Source: three-view drawing plus pictorial views. Frame: mm from the lowest corner of the part. Give positions to 0.01 mm unless a question says otherwise; leave off trailing zeros. Order: outer loops, then holes, each group sorted by start corner. A loop starts at its lowest first (then second) coordinate and runs counter-clockwise, first axis right, second up. Notation, with made-up numbers: (66.5, 85.25) -> (74.5, 85.25) arc R25 cw to (74.5, 120.25) -> close; hole circle Ø4 at (14, 84.5). An arc over 180 degrees is marked (long way). Answer in a Markdown table with one row per item. Add a question column.
Q1. Pull-direction query (X, two-part tool) for the marked faces 1, 2 and 3; classes: +X half, -X half, draft (parallel to the pull), parting line (faces both ways), or undercut.
Q2. Cut plane A-A on z = 40. Return the cut outline in (x, y).
Q3. Line query: line 1 along X through (y, z) = (2.8, 40); line 2 along X through (y, z) = (22, 40). Output: solid intervals per line, ascending. Write a range as from..to.
Q4. Cut plane C-C on y = 10.5. Return the cut outline in (x, z), and give its area (3 significant figures).
Q5. Cut plane B-B on x = 40. Return the cut outline in (y, z), and give its area (3 significant figures).
Q6. Cut plane D-D on x = 29.5. Return the cut outline in (y, z), and give its area (3 significant figures).
Q7. Contact query for flat-ended pins moving along their axis: P1, Ø5, axis at x = 55.5, y = 9.5, coming from the +Z side; P2, Ø2, axis at x = 49.5, y = 31, coming from the -Z side; P3, Ø1, axis at x = 58, y = 24.5, coming from the -Z side; P4, Ø1, axis at x = 57, z = 28.5, coming from the -Y side. Output: stop coordinate, or through.
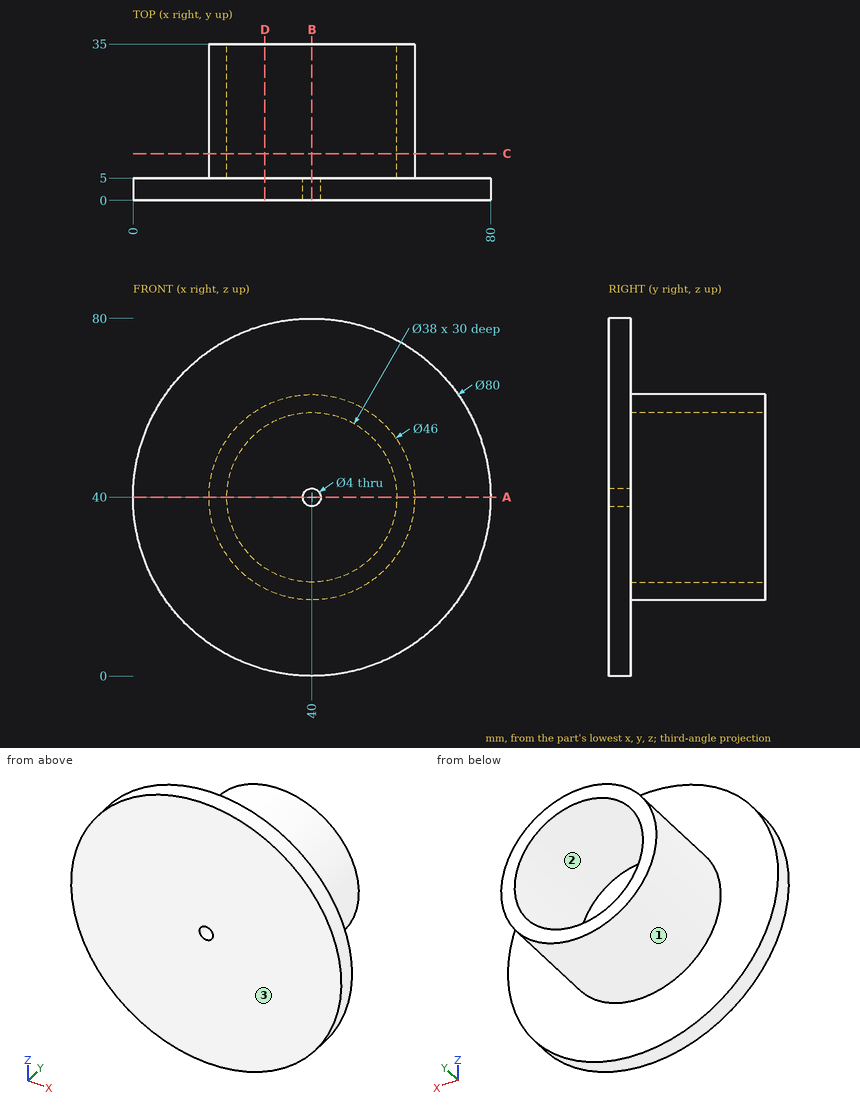
Completed:
| question | item | result |
|---|---|---|
| 1 | face 1 | parting line |
| 1 | face 2 | undercut |
| 1 | face 3 | draft |
| 2 | outline | (0, 0) -> (38, 0) -> (38, 5) -> (21, 5) -> (21, 35) -> (17, 35) -> (17, 5) -> (0, 5) -> close; (42, 0) -> (80, 0) -> (80, 5) -> (63, 5) -> (63, 35) -> (59, 35) -> (59, 5) -> (42, 5) -> close |
| 3 | line 1 | x = 0..38, 42..80 |
| 3 | line 2 | x = 17..21, 59..63 |
| 4 | outline | circle Ø46 at (40, 40); hole circle Ø38 at (40, 40) |
| 4 | area | 528 mm² |
| 5 | outline | (0, 0) -> (5, 0) -> (5, 17) -> (35, 17) -> (35, 21) -> (5, 21) -> (5, 38) -> (0, 38) -> close; (0, 42) -> (5, 42) -> (5, 59) -> (35, 59) -> (35, 63) -> (5, 63) -> (5, 80) -> (0, 80) -> close |
| 5 | area | 620 mm² |
| 6 | outline | (0, 1.4) -> (5, 1.4) -> (5, 19.54) -> (35, 19.54) -> (35, 24.16) -> (5, 24.16) -> (5, 55.84) -> (35, 55.84) -> (35, 60.46) -> (5, 60.46) -> (5, 78.6) -> (0, 78.6) -> close |
| 6 | area | 664 mm² |
| 7 | P1 | stops at z = 58.97 |
| 7 | P2 | stops at z = 18.63 |
| 7 | P3 | stops at z = 25.08 |
| 7 | P4 | stops at y = 0 |
